Check sheet for the modelled part. Datum: model origin and axes. Units: mm. Face numbers are marked on the shaded views. A direction names the side the tool comes from. Round coordinates to 2 decimals unless told otherwise and drop trailing zeros. Write each loop counter-clockwise with the first axis right and the second up, starting at its lowest first coordinate (ties: lowest second). Pieces come first, ordered by that corner, then holes. Notation, with made-up numbers: (-27, -16) - (11, -16) arc R23 cw to (11, 7) - close; hole circle Ø4 at (58, 32). An arc over 180 degrees is marked (long way). Answer as a JSON object with one key per item and string values. Group by question number.
Item 1: Sectioned sample at C-C on z = 0.75. Record the boundary of the cut face in (x, y), plus the area to 3 significant figures.
Item 2: Thickness scan on line 1 (Z direction, x = 0.2, y = 5); line 2 (Y direction, x = 0.8, z = -0.75). Record the ranges inside material, lowest first.
Item 3: Gauge pin test, flat ends, axial feed: P1, Ø1.5, axis at x = 1, y = 0.5, coming from the -Z side; P2, Ø0.9, axis at x = 2, z = 7, coming from the +Y side; P3, Ø0.9, axis at x = 1.5, y = 4.5, coming from the +Z side. Record the tip position at first contact, or that the pin passes through.
Item 4: Sectioned sample at B-B on y = -3.5. Record the boundary of the cut face in (x, z), plus the area to 3 significant figures.
Item 5: Set-up check for the marked faces 5 and 6: record each of +Z, -Z, +X, -X, +Y, -Y from which the full face is reachable in a straight line by a thin tool's end or side.
Item 6: Release check for a two-part mould opening along Z. For the marked faces 1, 2, 3 and 4 record: pulls with the +Z half, pulls with the -Z half, needs draft (parallel to the pull), parting line crosses it, or undercut.
Item 7: Sectioned sample at A-A on x = 0.7. Record the boundary of the cut face in (y, z).
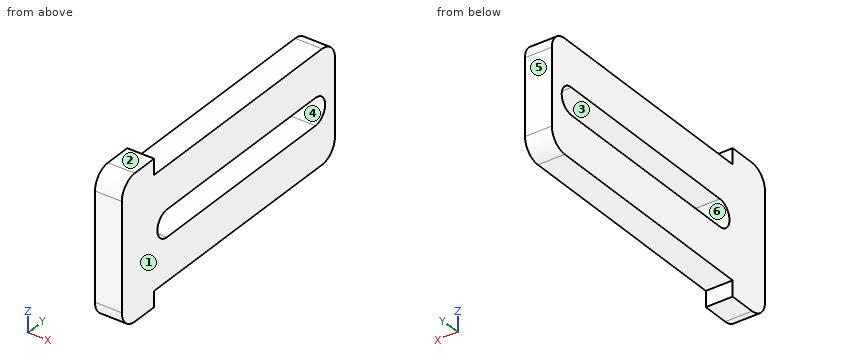
Autodesk Inventor part; units mm, degrees
ref_plane "YZ Plane" through (0, 0, 0) normal (1, 0, 0) x (0, 1, 0)
ref_plane "XZ Plane" through (0, 0, 0) normal (0, 1, 0) x (-1, 0, 0)
ref_plane "XY Plane" through (0, 0, 0) normal (0, 0, 1) x (1, 0, 0)
sketch "Sketch1" plane through (0, 0, 0) normal (1, 0, 0) x (0, 1, 0)
  line L0 (-11.5722, 7.9995) -> (-14.5722, 7.9995)
  line L1 (-16.5722, 5.9995) -> (-16.5722, -5.9996)
  line L2 (-14.5722, -7.9996) -> (-11.5722, -7.9996)
  line L3 (16.4278, 8.0004) -> (-16.5722, -7.9996) construction
  line L4 (-11.5722, 7.9995) -> (-11.5722, 6.2495)
  line L5 (-11.5722, 6.2495) -> (14.4277, 6.2507)
  line L6 (-11.5722, -6.2496) -> (14.4277, -6.2508)
  line L7 (-11.5722, 7.9995) -> (-11.5722, 6.2495)
  line L8 (-11.5722, -6.2496) -> (-11.5722, -7.9996)
  arc A0 (-14.5722, 7.9995) -> (-16.5722, 5.9995) centre (-14.5722, 5.9995) ccw
  arc A1 (-16.5722, -5.9996) -> (-14.5722, -7.9996) centre (-14.5722, -5.9996) ccw
  line L9 (-16.5722, 7.9995) -> (-3.1229, 1.4787) construction
  line L10 (-2.3653, 1.1122) -> (16.4278, -7.9996) construction
  arc A2 (13.4, -1.5001) -> (13.4, 1.4999) centre (13.4, -0.0001) ccw
  arc A3 (-9.6, 1.4999) -> (-9.6, -1.4996) centre (-9.5722, 0.0001) ccw
  line L11 (13.4, 1.4999) -> (-9.6, 1.4999)
  line L12 (-9.6, -1.4996) -> (13.4, -1.5001)
  line L13 (16.4278, 4.2507) -> (16.4278, -4.2508)
  arc A4 (16.4278, 4.2507) -> (14.4277, 6.2507) centre (14.4278, 4.2507) ccw
  arc A5 (14.4277, -6.2508) -> (16.4278, -4.2508) centre (14.4278, -4.2508) ccw
  point P0 (16.4278, 6.2508)
  point P1 (16.4278, -6.2509)
  dimension "d1" = 16
  dimension "d3" = 1.75
  dimension "d5" = 2
  dimension "d14" = 1.75
  dimension "d18" = 3
  dimension "d19" = 3
  dimension "d21" = 2
  dimension "d24" = 28
  dimension "d25" = 2
  dimension "d26" = 5
extrude "Extrusion3" add sketch "Sketch1" along normal blind 3
properties part number "Ga motor 1"
Completed:
{
 "1": {"outline": "(0, -16.57) - (3, -16.57) - (3, -10.87) - (0, -10.87) - close; (0, 14.7) - (3, 14.7) - (3, 16.43) - (0, 16.43) - close", "area": "22.3 mm²"},
 "2": {"line 1": "-6.25 to -1.5, 1.5 to 6.25", "line 2": "-16.57 to -10.87, 14.7 to 16.43"},
 "3": {"P1": "z = -6.25", "P2": "y = -11.57", "P3": "z = 6.25"},
 "4": {"outline": "(0, -6.25) - (3, -6.25) - (3, -1.5) - (0, -1.5) - close; (0, 1.5) - (3, 1.5) - (3, 6.25) - (0, 6.25) - close", "area": "28.5 mm²"},
 "5": {"face 5": "+Z, -Z, +X, -X, +Y", "face 6": "+X, -X"},
 "6": {"face 1": "needs draft", "face 2": "pulls with the +Z half", "face 3": "undercut", "face 4": "undercut"},
 "7": {"outline": "(-16.57, -6) arc R2 ccw to (-14.57, -8) - (-11.57, -8) - (-11.57, -6.25) - (14.43, -6.25) arc R2 ccw to (16.43, -4.25) - (16.43, 4.25) arc R2 ccw to (14.43, 6.25) - (-11.57, 6.25) - (-11.57, 8) - (-14.57, 8) arc R2 ccw to (-16.57, 6) - close; hole (-9.6, -1.5) - (13.4, -1.5) arc R1.5 ccw to (13.4, 1.5) - (-9.6, 1.5) arc R1.5 ccw to start"}
}
